Read the model definition and answer for the solid it produces. Units are mm, in the model's axes. Face numbers are marked on the shaded views. Give positions to 0.01 mm unless a question says otherwise; leave off trailing zeros. Write each loop counter-clockwise with the first axis right and the second up, starting at its lowest first coordinate (ties: lowest second). Pieces come first, ordered by that corner, then holes. Notation, with made-up numbers: (6, 49.5) - (59, 49.5) arc R15 cw to (59, 58.5) - close; hole circle Ø6 at (-35, 83). An arc over 180 degrees is marked (long way). Answer as CSV lines item,"result".
Autodesk Inventor part; units mm, degrees
ref_plane "YZ Plane" through (0, 0, 0) normal (1, 0, 0) x (0, 1, 0)
ref_plane "XZ Plane" through (0, 0, 0) normal (0, 1, 0) x (-1, 0, 0)
ref_plane "XY Plane" through (0, 0, 0) normal (0, 0, 1) x (1, 0, 0)
sketch "Szkic1" plane through (0, 0, 0) normal (0, 0, 1) x (1, 0, 0)
  line L0 (27, 15) -> (0, 15)
  line L1 (0, 0) -> (0, 15)
  line L2 (27, 0) -> (0, 0)
  line L3 (27, 0) -> (27, 15)
  circle A0 centre (13.5, 7.5) radius 2.5
  point P0 (27, 22.2042)
  dimension "d0" = 27
  dimension "d1" = 15
  dimension "d2" = 7.5
  dimension "d3" = 13.5
extrude "Wyciągnięcie proste1" add sketch "Szkic1" along normal blind 24
chamfer "Faza1" distance 1 angle 45 2 edges at (27, 15, 12) (0, 15, 12)
sketch "Szkic4" plane through (0, 0, 0) normal (0, -1, 0) x (1, 0, 0)
  line L0 (0, 0) -> (27, 0)
  line L1 (27, 0) -> (27, 24)
  line L2 (0, 24) -> (27, 24)
  line L3 (0, 0) -> (0, 24)
  point P0 (3.25, 4.15)
  point P1 (3.25, 15.85)
  point P2 (23.75, 4.15)
  point P3 (23.75, 15.85)
  dimension "d9" = 20.5
  dimension "d10" = 11.7
  dimension "d11" = 4.15
  dimension "d12" = 27
  dimension "d13" = 3.25
hole "Otwór1" at (3.25, 0, 4.15) at (3.25, 0, 15.85) at (23.75, 0, 4.15) at (23.75, 0, 15.85) direction (0, 1, 0) diameter 3 end through all
properties part number "3DP_ABS_Y_Axis_Tenioning_System_C_Sec_Filler"
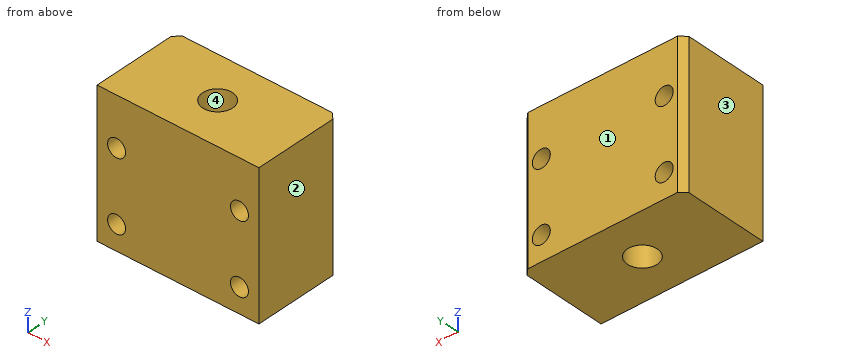
(1) The mould has two halves that part along X. Classify the marked faces 1, 2, 3 and 4: +X half, -X half, draft (parallel to the pull), parting line (faces both ways), or undercut.
Worked out:
face 1,"draft"
face 2,"+X half"
face 3,"-X half"
face 4,"undercut"
(2) A cutting plane is placed at A-A (z = 15.85). Write down the section's boundary in (x, y).
Worked out:
outline,"(0, 0) - (1.75, 0) - (1.75, 15) - (1, 15) - (0, 14) - close; (4.75, 0) - (22.25, 0) - (22.25, 15) - (4.75, 15) - close; (25.25, 0) - (27, 0) - (27, 14) - (26, 15) - (25.25, 15) - close; hole circle Ø5 at (13.5, 7.5)"
(3) Find the intervals of material crossed by L1, parallel to Z at x = 3.25, y = 10.5; L2, parallel to X at y = 11.75, z = 4.15; L3, parallel to X at y = 6.75, z = 4.15, in increasing order.
Worked out:
L1,"z = 0 to 2.65, 5.65 to 14.35, 17.35 to 24"
L2,"x = 0 to 1.75, 4.75 to 22.25, 25.25 to 27"
L3,"x = 0 to 1.75, 4.75 to 11.12, 15.88 to 22.25, 25.25 to 27"
(4) A cutting plane is placed at D-D (z = 11.75). Write down the section's boundary in (x, y).
Worked out:
outline,"(0, 0) - (27, 0) - (27, 14) - (26, 15) - (1, 15) - (0, 14) - close; hole circle Ø5 at (13.5, 7.5)"
(5) A cutting plane is placed at B-B (x = 13.5). Write down the section's boundary in (y, z).
Worked out:
outline,"(0, 0) - (5, 0) - (5, 24) - (0, 24) - close; (10, 0) - (15, 0) - (15, 24) - (10, 24) - close"
(6) A cutting plane is placed at C-C (y = 7.5). Write down the section's boundary in (x, z), and give its area (3 significant figures).
Worked out:
outline,"(0, 0) - (11, 0) - (11, 24) - (0, 24) - close; (16, 0) - (27, 0) - (27, 24) - (16, 24) - close; hole circle Ø3 at (3.25, 4.15); hole circle Ø3 at (3.25, 15.85); hole circle Ø3 at (23.75, 4.15); hole circle Ø3 at (23.75, 15.85)"
area,"500 mm^2"
